Build history of the part. All positions in model axes, mm. A direction names the side the tool comes from. Coordinates: 2 decimals unless noted, no trailing zeros. Loops run counter-clockwise (first coordinate to the right, second up) from the corner with the lowest first, then second, coordinate; pieces in that order, holes last.
Item 1: 3-axis set-ups, long thin cutter, end or side, ignore diameter. For faces 1 (the face through (3.233, -1.341, 0.246)), 2 (the face through (1.3, 0, 1)), 3 (the face through (0, -1.9, 2)), 4 (the face through (0, 1.3, 1)), 5 (the face through (-1.9, 0, 2)): which of +Z, -Z, +X, -X, +Y, -Y reach the whole face in a straight line?
Item 2: Cut at B-B (z = -0.5). List the corners of the cut face in (x, y), and give its area (3 significant figures).
Item 3: Drill centre lines: line 1 along Y through (x, z) = (0, 2.4); line 2 along Z through (x, y) = (-1.75, -0.75); line 3 along Y through (x, z) = (0, 1.05). Where is each one in solid material? Low to high.
Item 4: Cut at D-D (z = -3.25). List the corners of the cut face in (x, y), and give its area (4 significant figures).
Item 5: Mould opens along Y. For faces 6 (the face through (0, 0, 0.2)), 7 (the face through (0, -1.3, 1)), 8 (the face through (0, -2, 0.5)) say: released by +Y, released by -Y, zero draft, split by the parting line, or undercut.
Item 6: Cut at A-A (x = 0). List the corners of the cut face in (y, z).
Item 7: Flat gauge pins, fed straight in: pin 1 (6 mm diameter, centred on x = 4.5, y = 4.5, fed in from +Z); pin 2 (1.4 mm diameter, centred on x = 0.5, z = 2, fed in from -Y); pin 3 (1.5 mm diameter, centred on x = 2, y = 0, fed in from -Z). Where does each tip first touch, or does it go through?
from build123d import *

# Parameters (mm, degrees)
F0_W      = 12
F0_H      = 12
F0_R      = 3.5
F0_W_2    = 3.8
F0_H_2    = 3.8
F0_W_3    = 2.6
F0_H_3    = 2.6
F1_DEPTH  = 3.9
F2_DEPTH  = 0.5
F3_DEPTH  = 1.5
F4_R      = 1
F5_DEPTH  = 3
F6_W      = 3.8
F6_H      = 3.8
F6_W_2    = 2.6
F6_H_2    = 2.6
F7_DEPTH  = 1.7
F8_R      = 1
F9_DEPTH  = 3
F10_W     = 0.75
F10_H     = 3.05
F10_H_2   = 1.95
F12_DEPTH = 0.5
F13_R     = 0.49999
F11_W     = 0.75
F11_H     = 1.95
F11_H_2   = 3.05
F14_DEPTH = 0.5
F15_R     = 0.49999


# Not quite as in the source:
# - a fillet or chamfer is up to 0.001 mm smaller than in the source, because OpenCascade refuses the exact size


with BuildPart() as f1:
    # F0 (on Top) → F1 (new body)
    with BuildSketch(Plane.XY):
        Rectangle(F0_W, F0_H)
        Circle(F0_R, mode=Mode.SUBTRACT)
        Circle(F0_R)
        Rectangle(F0_W_2, F0_H_2, mode=Mode.SUBTRACT)
        Rectangle(F0_W_2, F0_H_2)
        Rectangle(F0_W_3, F0_H_3, mode=Mode.SUBTRACT)
        Rectangle(F0_W_3, F0_H_3)
    extrude(amount=-F1_DEPTH)

    # F0 (on Top) → F2 (join)
    with BuildSketch(Plane.XY):
        Circle(F0_R)
        Rectangle(F0_W_2, F0_H_2, mode=Mode.SUBTRACT)
        Rectangle(F0_W_2, F0_H_2)
        Rectangle(F0_W_3, F0_H_3, mode=Mode.SUBTRACT)
    extrude(amount=F2_DEPTH)

    # F0 (on Top) → F3 (join)
    with BuildSketch(Plane.XY):
        Rectangle(F0_W_3, F0_H_3)
    extrude(amount=F3_DEPTH)

    # F4 (on face) → F5 (cut)
    with BuildSketch(Plane.XY):
        Circle(F4_R)
    extrude(amount=-F5_DEPTH, mode=Mode.SUBTRACT)

    # F6 (on face) → F7 (join)
    with BuildSketch(Plane.XY.offset(1.5)):
        Rectangle(F6_W, F6_H)
        Rectangle(F6_W_2, F6_H_2, mode=Mode.SUBTRACT)
        Rectangle(F6_W_2, F6_H_2)
    extrude(amount=F7_DEPTH)

    # F8 (on face) → F9 (cut)
    with BuildSketch(Plane.XY.offset(3.2)):
        Circle(F8_R)
    extrude(amount=-F9_DEPTH, mode=Mode.SUBTRACT)

    # F10 (on face) → F12 (join)
    with BuildSketch(Plane.YZ.offset(6)):
        with Locations((-3.375, -5.425)):
            Rectangle(F10_W, F10_H)
        with Locations((-3.375, -2.925)):
            Rectangle(F10_W, F10_H_2)
        with Locations((3.375, -5.425)):
            Rectangle(F10_W, F10_H)
        with Locations((3.375, -2.925)):
            Rectangle(F10_W, F10_H_2)
    extrude(amount=F12_DEPTH)

    # F13 (radius 0.5 in the source; OpenCascade refuses exactly that, so slightly less here)
    f13_edges = [f1.edges().sort_by_distance(p)[0] for p in [
        (6.5, -3.375, -1.95),
        (6.5, 3.375, -1.95),
    ]]
    fillet(f13_edges, radius=F13_R)

    # F11 (on face) → F14 (join)
    with BuildSketch(Plane(origin=(-6, 0, 0), x_dir=(0, -1, 0), z_dir=(-1, 0, 0))):
        with Locations((3.375, -2.925)):
            Rectangle(F11_W, F11_H)
        with Locations((-3.375, -2.925)):
            Rectangle(F11_W, F11_H)
        with Locations((-3.375, -5.425)):
            Rectangle(F11_W, F11_H_2)
        with Locations((3.375, -5.425)):
            Rectangle(F11_W, F11_H_2)
    extrude(amount=F14_DEPTH)

    # F15 (radius 0.5 in the source; OpenCascade refuses exactly that, so slightly less here)
    f15_edges = [f1.edges().sort_by_distance(p)[0] for p in [
        (-6.5, 3.375, -1.95),
        (-6.5, -3.375, -1.95),
    ]]
    fillet(f15_edges, radius=F15_R)


solid = f1.part
Filled sheet:
1. face 1: +Z
1. face 2: +X, +Y, -Y
1. face 3: +Z, +X, -X, -Y
1. face 4: +X, -X, +Y
1. face 5: +Z, -X, +Y, -Y
2. outline: (-6, -6) - (6, -6) - (6, 6) - (-6, 6) - close; hole circle Ø2 at (0, 0)
2. area: 141 mm2
3. line 1: y = -1.9 to -1, 1 to 1.9
3. line 2: z = -3.9 to 0.5, 1.5 to 3.2
3. line 3: y = -1.3 to -1, 1 to 1.3
4. outline: (-6.5, -3.75) - (-6, -3.75) - (-6, -6) - (6, -6) - (6, -3.75) - (6.5, -3.75) - (6.5, -3) - (6, -3) - (6, 3) - (6.5, 3) - (6.5, 3.75) - (6, 3.75) - (6, 6) - (-6, 6) - (-6, 3.75) - (-6.5, 3.75) - (-6.5, 3) - (-6, 3) - (-6, -3) - (-6.5, -3) - close
4. area: 145.5 mm2
5. face 6: undercut
5. face 7: released by -Y
5. face 8: zero draft
6. outline: (-6, -3.9) - (6, -3.9) - (6, 0) - (3.5, 0) - (3.5, 0.5) - (1.3, 0.5) - (1.3, 1.5) - (1.9, 1.5) - (1.9, 3.2) - (1, 3.2) - (1, 0.2) - (-1, 0.2) - (-1, 3.2) - (-1.9, 3.2) - (-1.9, 1.5) - (-1.3, 1.5) - (-1.3, 0.5) - (-3.5, 0.5) - (-3.5, 0) - (-6, 0) - close; hole (-1, -3) - (1, -3) - (1, 0) - (-1, 0) - close
7. pin 1: stops at z = 0.5
7. pin 2: stops at y = -1.9
7. pin 3: stops at z = -3.9
